Source: CAD feature listing. Evaluate the final solid. Frame: model axes, mm. Face numbers are marked on the shaded views. A direction names the side the tool comes from. Give positions to 0.01 mm unless a question says otherwise; leave off trailing zeros. Order: outer loops, then holes, each group sorted by start corner. A loop starts at its lowest first (then second) coordinate and runs counter-clockwise, first axis right, second up. Notation, with made-up numbers: (75.25, 12.25) - (122.25, 12.25) arc R23 cw to (122.25, 43.25) - close; hole circle Ø10 at (73, 63.25). An arc over 180 degrees is marked (long way). Use CSV: the item, a comma, the result in double quotes.
```python
from build123d import *

# Parameters (mm, degrees)
SKETCH2_W           = 118.11
SKETCH2_H           = 92.71
BOSS_EXTRUDE2_DEPTH = 63.5
SHELL1_T            = -2.54
SKETCH3_R           = 6.985
CUT_EXTRUDE1_DEPTH  = 90.17
CUT_EXTRUDE2_REACH  = 120.11
SKETCH4_R           = 5.08
CUT_EXTRUDE3_REACH  = 120.11
SKETCH5_R           = 3.81


with BuildPart() as part:
    # Sketch2 → Boss-Extrude2 (new body)
    with BuildSketch(Plane(origin=(0, 0, 0), x_dir=(1, 0, 0), z_dir=(0, 1, 0))):
        Rectangle(SKETCH2_W, SKETCH2_H)
    extrude(amount=BOSS_EXTRUDE2_DEPTH)

    # Shell1
    shell1_openings = [part.faces().sort_by_distance(p)[0] for p in [
        (0, 63.5, 0),
    ]]
    offset(amount=SHELL1_T, openings=shell1_openings, kind=Kind.INTERSECTION)

    # Sketch3 → Cut-Extrude1 (cut)
    with BuildSketch(Plane.XY.offset(46.355)):
        with Locations((20.955, 9.652)):
            Circle(SKETCH3_R)
    extrude(amount=-CUT_EXTRUDE1_DEPTH, mode=Mode.SUBTRACT)

    # Sketch4 → Cut-Extrude2 (cut, up to next)
    with BuildSketch(Plane.ZY.offset(59.055), mode=Mode.PRIVATE) as cut_extrude2_sk1:
        with Locations((26.035, 53.34)):
            Circle(SKETCH4_R)
    cut_extrude2_tool1 = extrude(cut_extrude2_sk1.sketch, amount=-CUT_EXTRUDE2_REACH, mode=Mode.PRIVATE) & part.part
    add(cut_extrude2_tool1.solids().sort_by_distance((-59.055, 53.34, 26.035))[0], mode=Mode.SUBTRACT)

    # Sketch5 → Cut-Extrude3 (cut, up to next)
    with BuildSketch(Plane.ZY.offset(59.055), mode=Mode.PRIVATE) as cut_extrude3_sk1:
        with Locations((-20.955, 53.34)):
            Circle(SKETCH5_R)
    cut_extrude3_tool1 = extrude(cut_extrude3_sk1.sketch, amount=-CUT_EXTRUDE3_REACH, mode=Mode.PRIVATE) & part.part
    add(cut_extrude3_tool1.solids().sort_by_distance((-59.055, 53.34, -20.955))[0], mode=Mode.SUBTRACT)


solid = part.part
```
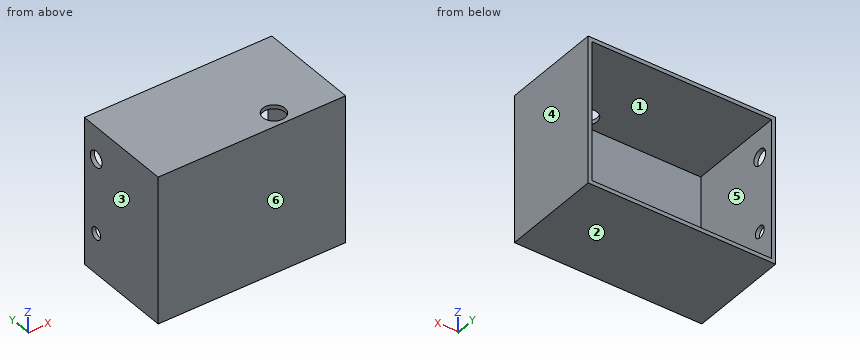
Item 1: Section A-A on y = 30. Return the cut outline in (x, z) (3 decimals), then the cut area to 3 significant figures.
Filled in:
outline,"(-59.055, -46.355) - (59.055, -46.355) - (59.055, 46.355) - (-59.055, 46.355) - close; hole (-56.515, -43.815) - (56.515, -43.815) - (56.515, 43.815) - (-56.515, 43.815) - close"
area,"1,050 mm2"
Item 2: Set-up query: the marked faces 1 and 2. Return all of +Z, -Z, +X, -X, +Y, -Y with unobstructed straight access to the full face (end or side cutting, diameter ignored); none if empty.
Filled in:
face 1,"+Y"
face 2,"-Z, +X, -X, +Y, -Y"
Item 3: Section D-D on z = 9.5. Return the cut outline in (x, y) (3 decimals).
Filled in:
outline,"(-59.055, 0) - (59.055, 0) - (59.055, 63.5) - (56.515, 63.5) - (56.515, 2.54) - (-56.515, 2.54) - (-56.515, 63.5) - (-59.055, 63.5) - close"
Item 4: Material intervals for line 1 (X direction, y = 57, z = -11.5) (3 decimals); line 2 (Z direction, x = -17, y = 53.5) (3 decimals); line 3 (Y direction, x = -45, z = -31.5), sorted ascending. Write a range as from..to.
Filled in:
line 1,"x = -59.055..-56.515, 56.515..59.055"
line 2,"z = -46.355..-43.815, 43.815..46.355"
line 3,"y = 0..2.54"
Item 5: Section C-C on y = 53.34. Return the cut outline in (x, z) (3 decimals).
Filled in:
outline,"(-59.055, -46.355) - (59.055, -46.355) - (59.055, 46.355) - (-59.055, 46.355) - (-59.055, 31.115) - (-56.515, 31.115) - (-56.515, 43.815) - (56.515, 43.815) - (56.515, -43.815) - (-56.515, -43.815) - (-56.515, -24.765) - (-59.055, -24.765) - close; (-59.055, -17.145) - (-56.515, -17.145) - (-56.515, 20.955) - (-59.055, 20.955) - close"
Item 6: Section B-B on z = 22.5. Return the cut outline in (x, y) (3 decimals).
Filled in:
outline,"(-59.055, 0) - (59.055, 0) - (59.055, 63.5) - (56.515, 63.5) - (56.515, 2.54) - (-56.515, 2.54) - (-56.515, 49.692) - (-59.055, 49.692) - close; (-59.055, 56.988) - (-56.515, 56.988) - (-56.515, 63.5) - (-59.055, 63.5) - close"
Item 7: First-contact query: pin 1 (13 mm diameter, centred on y = 53.34, z = 26.035, fed in from -X) (3 decimals); pin 2 (1 mm diameter, centred on x = 21.5, z = -26, fed in from +Y); pin 3 (4.5 mm diameter, centred on y = 53.34, z = -20.955, fed in from -X) (3 decimals). Flat tips, straight axial feed; report the tip coordinate or a pass-through.
Filled in:
pin 1,"stops at x = -59.055"
pin 2,"stops at y = 2.54"
pin 3,"stops at x = 56.515"
Item 8: Mould query, pull axis X, two halves, no side actions, for the marked faces 3, 4, 5 and 6. Classes: released by +X, released by -X, zero draft, split by the parting line, or undercut.
Filled in:
face 3,"released by -X"
face 4,"released by +X"
face 5,"undercut"
face 6,"zero draft"
